Part print with two shaded views. Sizes in mm from the minimum x, y, z corner. Give positions to 0.01 mm unless a question says otherwise; leave off trailing zeros. Write each loop counter-clockwise with the first axis right and the second up, starting at its lowest first coordinate (ties: lowest second). Pieces come first, ordered by that corner, then holes.
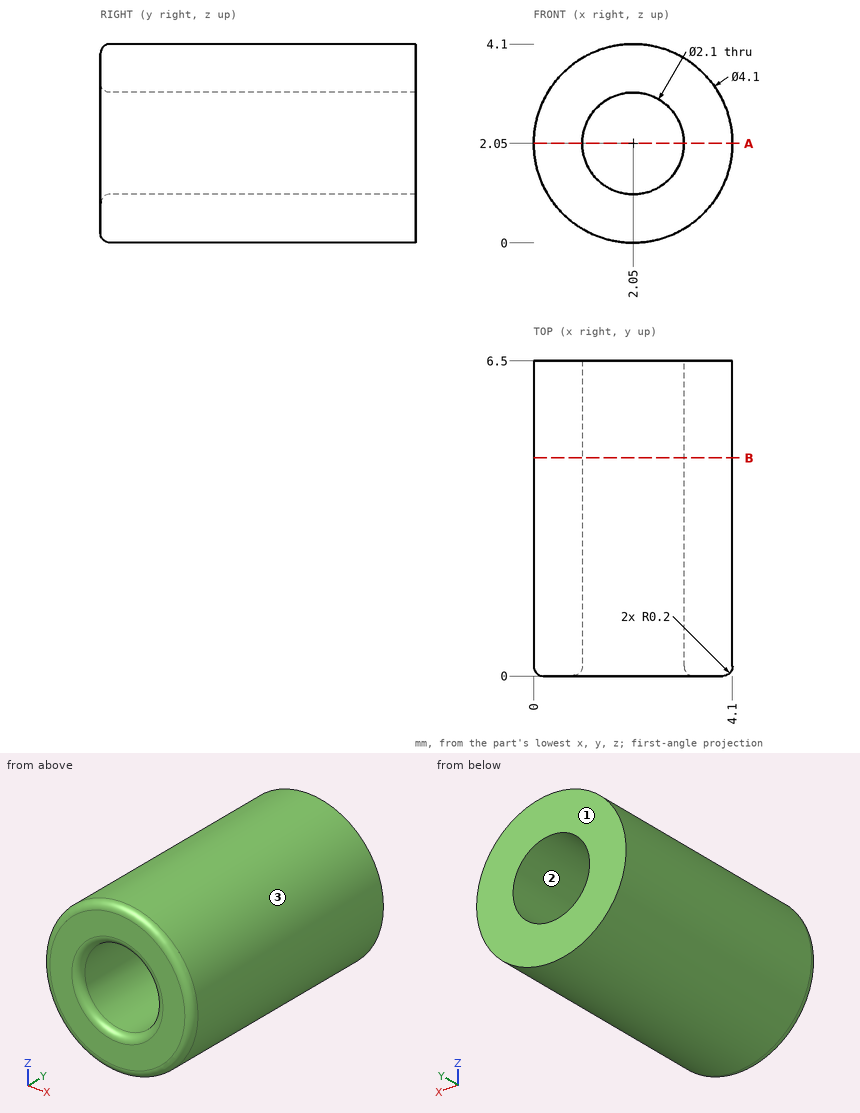
(1) Saw through at B-B, the plane y = 4.5. List the corners of the cut face in (x, z), plus the area to 3 significant figures.
(2) Saw through at A-A, the plane z = 2.05. List the corners of the cut face in (x, y).
(3) Probe line 1 (X direction, y = 4, z = 2.05); line 2 (Z direction, x = 2.7, y = 4.5). List the from-to ranges inside material, lowest first.
(4) Mould opens along Z. For the marked faces 1, 2 and 3 say: +Z half, -Z half, draft (parallel to the pull), parting line (faces both ways), or undercut.
(5) Drop a flat-ended pin along its axis: pin 1 (1.3 mm diameter, centred on x = 2.05, z = 2.05, fed in from -Y). Give the stop position or say it passes through.
Computed values:
1. outline: circle Ø4.1 at (2.05, 2.05); hole circle Ø2.1 at (2.05, 2.05)
1. area: 9.74 mm2
2. outline: (0, 0.2) arc R0.2 ccw to (0.2, 0) - (0.8, 0) arc R0.2 ccw to (1, 0.2) - (1, 6.5) - (0, 6.5) - close; (3.1, 0.2) arc R0.2 ccw to (3.3, 0) - (3.9, 0) arc R0.2 ccw to (4.1, 0.2) - (4.1, 6.5) - (3.1, 6.5) - close
3. line 1: x = 0 to 1, 3.1 to 4.1
3. line 2: z = 0.11 to 1.23, 2.87 to 3.99
4. face 1: draft
4. face 2: undercut
4. face 3: parting line
5. pin 1: passes through
